```python
from build123d import *

# Parameters (mm, degrees)
SKETCH2_W           = 20
SKETCH2_H           = 20
BOSS_EXTRUDE1_DEPTH = 20
SKETCH3_W           = 20
SKETCH3_H           = 19
CUT_EXTRUDE1_DEPTH  = 19
SKETCH4_R           = 5
CUT_EXTRUDE2_DEPTH  = 17.5
BOSS_EXTRUDE2_DEPTH = 4
SKETCH10_R          = 2.5
CUT_EXTRUDE3_DEPTH  = 2
CUT_EXTRUDE4_DEPTH  = 2


with BuildPart() as part:
    # Sketch2 → Boss-Extrude1 (new body)
    with BuildSketch(Plane.XY):
        with Locations((10, 10)):
            Rectangle(SKETCH2_W, SKETCH2_H)
    extrude(amount=BOSS_EXTRUDE1_DEPTH)

    # Sketch3 → Cut-Extrude1 (cut)
    with BuildSketch(Plane.XY.offset(20)):
        with Locations((10, 9.5)):
            Rectangle(SKETCH3_W, SKETCH3_H)
    extrude(amount=-CUT_EXTRUDE1_DEPTH, mode=Mode.SUBTRACT)

    # Sketch4 → Cut-Extrude2 (cut)
    with BuildSketch(Plane.XZ.offset(-19)):
        with Locations((10, 10)):
            Circle(SKETCH4_R)
    extrude(amount=-CUT_EXTRUDE2_DEPTH, mode=Mode.SUBTRACT)

    # Sketch6 → Boss-Extrude2 (add)
    with BuildSketch(Plane.XY.offset(1)):
        with BuildLine():
            Line((7.5, 3), (7.5, 8))
            ThreePointArc((7.5, 8), (10, 10.5), (12.5, 8))
            Line((12.5, 8), (12.5, 3))
            Line((12.5, 3), (14.603533184, 3))
            Line((14.603533184, 3), (14.603533184, 8))
            ThreePointArc((14.603533184, 8), (10, 12.603533184), (5.396466816, 8))
            Line((5.396466816, 8), (5.396466816, 3))
            Line((5.396466816, 3), (7.5, 3))
        make_face()
    extrude(amount=BOSS_EXTRUDE2_DEPTH)

    # Sketch10 → Cut-Extrude3 (cut, through all)
    with BuildSketch(Plane.XY.offset(1)):
        with Locations((5, 15)):
            Circle(SKETCH10_R)
        with Locations((15, 15)):
            Circle(SKETCH10_R)
    extrude(amount=-CUT_EXTRUDE3_DEPTH, mode=Mode.SUBTRACT)

    # Sketch11 → Cut-Extrude4 (cut)
    with BuildSketch(Plane(origin=(0, 20, 0), x_dir=(1, 0, 0), z_dir=(0, 1, 0))):
        with BuildLine():
            Line((7.5, -5.669872981), (7.5, -2.669872981))
            Line((7.5, -2.669872981), (12.5, -2.669872981))
            Line((12.5, -2.669872981), (12.5, -5.669872981))
            ThreePointArc((12.5, -5.669872981), (10, -5), (7.5, -5.669872981))
        make_face()
    extrude(amount=-CUT_EXTRUDE4_DEPTH, mode=Mode.SUBTRACT)


solid = part.part
```
Geometry check sheet. Reference: the model listing, model coordinates, mm. A direction names the side the tool comes from. Coordinates: 2 decimals unless noted, no trailing zeros. Write each loop counter-clockwise with the first axis right and the second up, starting at its lowest first coordinate (ties: lowest second). Pieces come first, ordered by that corner, then holes. Notation, with made-up numbers: M 75.25,53 L 91.25,53 A15 ccw 91.25,57 Z; hole C 73.5,35.25 d2. An arc over 180 degrees is marked long. Answer as a JSON object with one key per item and string values.
1. Section check A-A, the plane y = 15. Enter the section's corners in (x, z), plus the area to 3 significant figures.
Answers below:
{"outline": "M 0,0 L 2.5,0 L 2.5,1 L 0,1 Z; M 7.5,0 L 12.5,0 L 12.5,1 L 7.5,1 Z; M 17.5,0 L 20,0 L 20,1 L 17.5,1 Z", "area": "10.0 mm²"}
2. Go/stop test with flat-tipped pins: pin 1 Ø12 at (x, z) = (17.5, 13) entering from -Y; pin 2 Ø0.6 at (x, z) = (13.5, 2.5) entering from -Y; pin 3 Ø10 at (x, y) = (9.5, 9) entering from +Z. Record where each tip stops, or that it passes through.
Answers below:
{"pin 1": "stops at y = 19", "pin 2": "stops at y = 3", "pin 3": "stops at z = 5"}
3. Section check D-D, the plane x = 13.25. Enter the section's corners in (y, z), plus the area to 3 significant figures.
Answers below:
{"outline": "M 0,0 L 13.21,0 L 13.21,1 L 11.26,1 L 11.26,5 L 3,5 L 3,1 L 0,1 Z; M 16.79,0 L 20,0 L 20,6.2 L 19,6.2 L 19,1 L 16.79,1 Z; M 19,13.8 L 20,13.8 L 20,20 L 19,20 Z", "area": "60.9 mm²"}
4. Tool access check on faces 5 (the cylindrical face through (10.101, 12.602, 2.972)), 6 (the flat face through (14, 3, 3)), 7 (the cylindrical face through (9.9, 10.5, 3)). Record the directions out of +Z, -Z, +X, -X, +Y, -Y that give a thin tool (end or side, any length) a straight path to the whole face; none if there is none.
Answers below:
{"face 5": "+Z", "face 6": "+Z, +X, -X, -Y", "face 7": "+Z, -Y"}
5. Section check C-C, the plane z = 10. Enter the section's corners in (x, y).
Answers below:
{"outline": "M 0,19 L 5,19 L 5,20 L 0,20 Z; M 15,19 L 20,19 L 20,20 L 15,20 Z"}
6. Section check B-B, the plane x = 10. Enter the section's corners in (y, z).
Answers below:
{"outline": "M 0,0 L 20,0 L 20,2.67 L 19,2.67 L 19,1 L 12.6,1 L 12.6,5 L 10.5,5 L 10.5,1 L 0,1 Z; M 19,15 L 20,15 L 20,20 L 19,20 Z"}
7. Scan lines: L1, parallel to X at y = 19.35, z = 10; L2, parallel to Z at x = 10, y = 19.65; L3, parallel to X at y = 6.5, z = 4. Record each from-to range of solid material in increasing order.
Answers below:
{"L1": "x = 0 to 5, 15 to 20", "L2": "z = 0 to 2.67, 15 to 20", "L3": "x = 5.4 to 7.5, 12.5 to 14.6"}
8. Draft check along Y on faces 1 (the flat face through (10, 10, 1)), 2 (the flat face through (20, 14.4, 0.3)), 3 (the flat face through (6, 3, 3)), 4 (the cylindrical face through (7.31, 14.04, 0.51)). Enter one of: released by +Y, released by -Y, zero draft, split by the parting line, or undercut.
Answers below:
{"face 1": "undercut", "face 2": "zero draft", "face 3": "released by -Y", "face 4": "undercut"}
